For this review, take the finished solid that the model builds, in its own axes (mm). Round coordinates to 2 decimals unless told otherwise and drop trailing zeros. Write each loop counter-clockwise with the first axis right and the second up, starting at its lowest first coordinate (ties: lowest second). Pieces come first, ordered by that corner, then holes. Notation, with made-up numbers: M -23.5,76 L 2.5,76 A30 cw 2.5,112 Z; hole C 49,84 d1. An arc over 180 degrees is marked long. Answer in a Markdown table with one row per item.
```python
from build123d import *

# Parameters (mm, degrees)
STOCK_BATTERY_BASE_1_DEPTH   = 7.5
STOCK_BATTERY_BASE_1_2_DEPTH = 4.5
BOSS_EXTRUDE1_DEPTH          = 2.5
SKETCH2_W                    = 2.5
SKETCH2_H                    = 97.061474856
BOSS_EXTRUDE2_DEPTH          = 7


# Read off the part's stored shape, not the designer's step: Stock-battery base-1
with BuildPart() as part:
    # Stock-battery base-1 outline → Stock-battery base-1 (new body)
    with BuildSketch(Plane.XY):
        with BuildLine():
            Line((16.459100066, -58.832087736), (16.459100066, 43.22938712))
            Line((16.459100066, 43.22938712), (0.459100066, 44.038083245))
            Line((0.459100066, 44.038083245), (0.459100066, 47.61329436))
            Line((0.459100066, 47.61329436), (-75.963345356, 51.475952827))
            add(Edge.make_bspline(
                [(-75.963345356, 51.475952827), (-76.969760945, 51.385311169), (-77.956664013, 51.213742336), (-79.395866789, 50.78571401), (-79.86970863, 50.613871194), (-80.796837185, 50.204577199), (-81.240590365, 49.971323111), (-82.089787414, 49.449496549), (-82.495246976, 49.160946736), (-83.271465049, 48.533739024), (-83.643007435, 48.194375714), (-84.708444042, 47.116795042), (-85.333215001, 46.343374139), (-86.491296884, 44.737676097), (-87.023827607, 43.904896882), (-88.044872363, 42.211012893), (-88.533034054, 41.34968138), (-89.982900727, 38.756279626), (-90.93240726, 37.013628654), (-92.999467157, 33.650383947), (-94.114586107, 32.031232641), (-95.60337212, 30.287705281), (-95.819744565, 30.042891916), (-96.040899934, 29.801740739)],
                knots=[0, 0, 0, 0, 0.0625, 0.0625, 0.09375, 0.09375, 0.125, 0.125, 0.15625, 0.15625, 0.1875, 0.1875, 0.25, 0.25, 0.3125, 0.3125, 0.375, 0.375, 0.5, 0.5, 0.625, 0.625, 0.645748558, 0.645748558, 0.645748558, 0.645748558], degree=3))
            Line((-96.040899934, 29.801740739), (-101.040899934, 29.801740739))
            Line((-101.040899934, 29.801740739), (-101.040899934, -41.829259963))
            Line((-101.040899934, -41.829259963), (-96.040899934, -41.829259963))
            add(Edge.make_bspline(
                [(-96.040899934, -41.829259963), (-95.798899268, -42.093160096), (-95.56197213, -42.362136183), (-94.03954966, -44.156758027), (-92.923608678, -45.792412437), (-90.858487716, -49.170948695), (-89.911065512, -50.914960796), (-88.457766632, -53.51029646), (-87.967520262, -54.371999904), (-86.940892781, -56.06392928), (-86.404912323, -56.894254814), (-85.530671439, -58.091259413), (-85.227414802, -58.482089731), (-84.588818098, -59.241614046), (-84.254184704, -59.609132259), (-83.204929916, -60.651600397), (-82.440569541, -61.270576891), (-81.160629249, -62.042718444), (-80.719255742, -62.269433113), (-79.817314106, -62.660888928), (-79.3554021, -62.826549047), (-77.940467092, -63.243286827), (-76.954208328, -63.414201398), (-75.963345356, -63.503442328)],
                knots=[0.352672192, 0.352672192, 0.352672192, 0.352672192, 0.375, 0.375, 0.5, 0.5, 0.625, 0.625, 0.6875, 0.6875, 0.75, 0.75, 0.78125, 0.78125, 0.8125, 0.8125, 0.875, 0.875, 0.90625, 0.90625, 0.9375, 0.9375, 1, 1, 1, 1], degree=3))
            Line((-75.963345356, -63.503442328), (16.459100066, -58.832087736))
        make_face()
    extrude(amount=STOCK_BATTERY_BASE_1_DEPTH)

    # Stock-battery base-1 2 outline → Stock-battery base-1 2 (add)
    with BuildSketch(Plane.XY):
        Polygon((16.459100066, 43.22938712), (16.459100066, 46.804598235), (0.459100066, 47.61329436), (0.459100066, 44.038083245), align=None)
    extrude(amount=STOCK_BATTERY_BASE_1_2_DEPTH)

    # Sketch1 → Boss-Extrude1 (add)
    with BuildSketch(Plane(origin=(16.459100066, 0, 0), x_dir=(0, 0, -1), z_dir=(1, 0, 0))):
        Polygon((0, -58.832087736), (0, 46.804598235), (-4.5, 46.804598235), (-4.5, 43.22938712), (-7.5, 43.22938712), (-7.5, -58.832087736), align=None)
    extrude(amount=BOSS_EXTRUDE1_DEPTH)

    # Sketch2 → Boss-Extrude2 (add)
    with BuildSketch(Plane(origin=(18.959100066, 0, 0), x_dir=(0, 0, -1), z_dir=(1, 0, 0))):
        with Locations((-3.75, -7.801350308)):
            Rectangle(SKETCH2_W, SKETCH2_H)
    extrude(amount=BOSS_EXTRUDE2_DEPTH)


solid = part.part
```
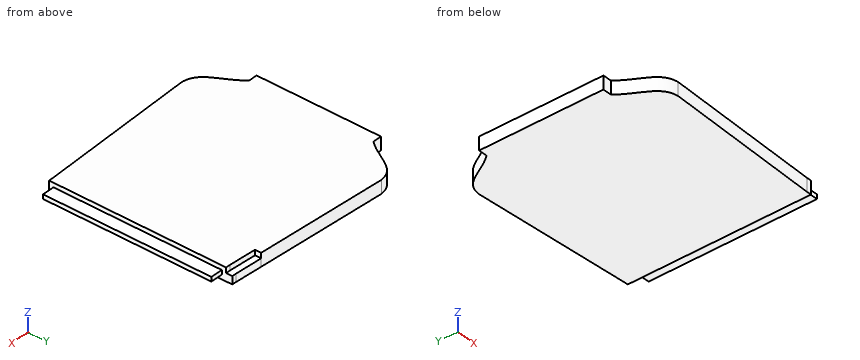
Q1. Take a section at A-A (y = -31). State the section outline as (x, z) points, then the cut area to 4 significant figures.
Found:
| item | result |
|---|---|
| outline | M -101.04,0 L 18.96,0 L 18.96,2.5 L 25.96,2.5 L 25.96,5 L 18.96,5 L 18.96,7.5 L -101.04,7.5 Z |
| area | 917.5 mm² |
Q2. For probe 1 along X at (y, z) = (-6, 2.25); probe 2 along X at (y, z) = (40.5, 0.75); probe 3 along Y at (x, z) = (-56, 3), list the stretches that pass through material, from the lowest coordinate up.
Found:
| item | result |
|---|---|
| probe 1 | -101.04 to 18.96 |
| probe 2 | -89.01 to 18.96 |
| probe 3 | -62.49 to 50.47 |
Q3. Take a section at C-C (x = -42). State the section outline as (y, z) points, then the cut area to 3 significant figures.
Found:
| item | result |
|---|---|
| outline | M -61.79,0 L 49.76,0 L 49.76,7.5 L -61.79,7.5 Z |
| area | 837 mm² |
Q4. Insertion check: P1, Ø2, axis at x = 23, z = 3, coming from the +Y side; P2, Ø2, axis at x = 17.5, z = 2, coming from the +Y side; P3, Ø1.5, axis at x = -98.5, z = 4, coming from the +Y side. Each pin has a flat end and moves straight along its axis. Give the tip position at first contact, or say it passes through.
Found:
| item | result |
|---|---|
| P1 | y = 40.73 |
| P2 | y = 46.8 |
| P3 | y = 29.8 |
Q5. Take a section at B-B (x = 11.5). State the section outline as (y, z) points, then the cut area to 3 significant figures.
Found:
| item | result |
|---|---|
| outline | M -59.08,0 L 47.06,0 L 47.06,4.5 L 43.48,4.5 L 43.48,7.5 L -59.08,7.5 Z |
| area | 785 mm² |
